Part print with two shaded views. Sizes in mm from the minimum x, y, z corner. Round coordinates to 2 decimals unless told otherwise and drop trailing zeros. Write each loop counter-clockwise with the first axis right and the second up, starting at its lowest first coordinate (ties: lowest second). Pieces come first, ordered by that corner, then holes.
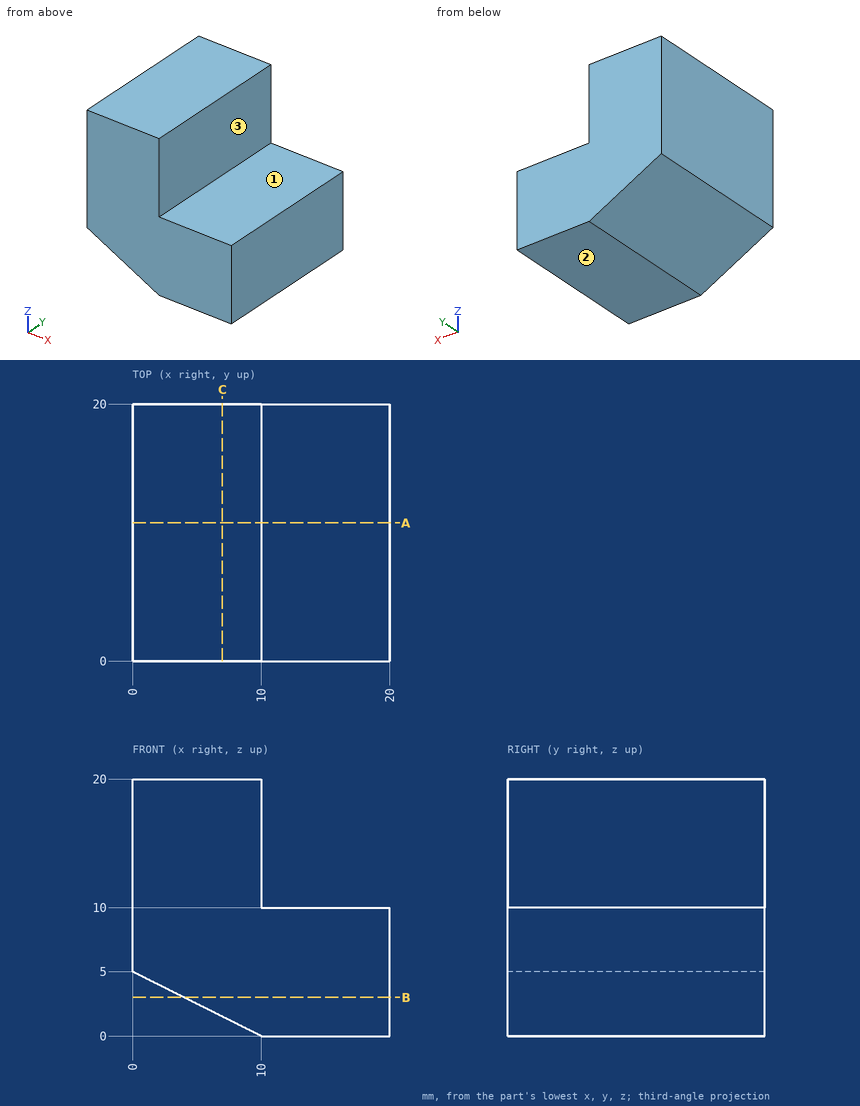
Q1. Drop flat-ended pins along their axis: pin 1 (1 mm diameter, centred on x = 12, y = 18, fed in from +Z); pin 2 (8 mm diameter, centred on x = 10.5, z = 11.5, fed in from +Y); pin 3 (1 mm diameter, centred on x = 3, y = 7.5, fed in from -Z). Give the stop position or say it passes through.
Values follow:
pin 1: stops at z = 10
pin 2: stops at y = 20
pin 3: stops at z = 3.25
Q2. Cut at A-A on y = 10.75. Write the cut outline in (x, z), plus the area to 3 significant figures.
Values follow:
outline: (0, 5) - (10, 0) - (20, 0) - (20, 10) - (10, 10) - (10, 20) - (0, 20) - close
area: 275 mm2
Q3. Cut at C-C on x = 7. Write the cut outline in (y, z).
Values follow:
outline: (0, 1.5) - (20, 1.5) - (20, 20) - (0, 20) - close
Q4. Mould opens along Z. For the marked faces 1, 2 and 3 say: +Z half, -Z half, draft (parallel to the pull), parting line (faces both ways), or undercut.
Values follow:
face 1: +Z half
face 2: -Z half
face 3: draft
Q5. Wall check: L1, parallel to X at y = 14.75, z = 13.5; L2, parallel to X at y = 8.5, z = 1. Give the ranges that are in metal, low to high.
Values follow:
L1: x = 0 to 10
L2: x = 8 to 20
Q6. Cut at B-B on z = 3. Write the cut outline in (x, y), plus the area to 3 significant figures.
Values follow:
outline: (4, 0) - (20, 0) - (20, 20) - (4, 20) - close
area: 320 mm2
